For this review, take the finished solid that the model builds, in its own axes (mm). A direction names the side the tool comes from. Give positions to 0.01 mm unless a question says otherwise; leave off trailing zeros. Order: outer loops, then holes, each group sorted by start corner. A loop starts at its lowest first (then second) coordinate and runs counter-clockwise, first axis right, second up.
from build123d import *

# Parameters (mm, degrees)
SKETCH1_R             = 15
BOSS_EXTRUDE1_DEPTH   = 2
SKETCH2_W             = 12
SKETCH2_H             = 12
BOSS_EXTRUDE2_DEPTH   = 15
SKETCH3_R             = 2.5
CUT_EXTRUDE1_DEPTH    = 30.849623113
SKETCH4_R             = 10
BOSS_EXTRUDE3_DEPTH   = 30
FILLET1_R             = 5
SKETCH5_R             = 1.5
BOSS_EXTRUDE4_DEPTH   = 20
SKETCH7_R             = 0.5
BODY_MOVE_COPY2_ANGLE = 90


with BuildPart() as part:
    # Sketch1 → Boss-Extrude1 (new body)
    with BuildSketch(Plane.XY):
        Circle(SKETCH1_R)
    extrude(amount=-BOSS_EXTRUDE1_DEPTH)

    # Sketch2 → Boss-Extrude2 (add)
    with BuildSketch(Plane.XY):
        Rectangle(SKETCH2_W, SKETCH2_H)
    extrude(amount=BOSS_EXTRUDE2_DEPTH)

    # Sketch3 → Cut-Extrude1 (cut, through all)
    with BuildSketch(Plane(origin=(6, 0, 0), x_dir=(0, 0, -1), z_dir=(1, 0, 0))):
        with Locations(Location((-7.5, 0, 0), (0, 0, 90))):
            Circle(SKETCH3_R)
    extrude(amount=-CUT_EXTRUDE1_DEPTH, mode=Mode.SUBTRACT)

    # Sketch4 → Boss-Extrude3 (add)
    with BuildSketch(Plane(origin=(0, 0, -2), x_dir=(-1, 0, 0), z_dir=(0, 0, -1))):
        with Locations(Location((0, 0, 0), (0, 0, 180))):
            Circle(SKETCH4_R)
    extrude(amount=BOSS_EXTRUDE3_DEPTH)

    # Fillet1
    fillet1_edges = [part.edges().sort_by_distance(p)[0] for p in [
        (-10, 0, -32),
    ]]
    fillet(fillet1_edges, radius=FILLET1_R)

    # Sketch5 → Boss-Extrude4 (add)
    with BuildSketch(Plane(origin=(0, 0, -32), x_dir=(-1, 0, 0), z_dir=(0, 0, -1))):
        Circle(SKETCH5_R)
    extrude(amount=BOSS_EXTRUDE4_DEPTH)

    # Sketch7 → Loft2 section 0
    with BuildSketch(Plane(origin=(0, 0, -52), x_dir=(-1, 0, 0), z_dir=(0, 0, -1)), mode=Mode.PRIVATE) as loft2_s0:
        Circle(SKETCH7_R)
    loft([Vertex(0, 0, -54.75), loft2_s0.sketch])


with BuildPart() as part_1:
    # Body-Move/Copy1: moved
    add(part.part.moved(Location((0, 0, 52))))


with BuildPart() as part_2:
    # Body-Move/Copy2: moved
    add(part_1.part.rotate(Axis((0, 0, 0), (0, 1, 0)), BODY_MOVE_COPY2_ANGLE))


solid = part_2.part
1) We need section A-A on x = 59.5. Give the boundary of the cut face in (y, z).
Answer sheet:
outline: (-6, -6) - (-2.5, -6) - (-2.5, 6) - (-6, 6) - close; (2.5, -6) - (6, -6) - (6, 6) - (2.5, 6) - close
2) We need section B-B on x = 13.5. Give the boundary of the cut face in (y, z).
Answer sheet:
outline: circle Ø3 at (0, 0)
3) We need section D-D on x = 35. Give the boundary of the cut face in (y, z), then the cut area to 3 significant figures.
Answer sheet:
outline: circle Ø20 at (0, 0)
area: 314 mm2
4) Tool access review of faces 1 (the face through (59, 6, 0)), 2 (the face through (59, -6, 0)), 3 (the face through (59, 3, -6)), 4 (the face through (20, -1.2, 1.2)): name each direction out of +Z, -Z, +X, -X, +Y, -Y from which nothing blocks a thin tool from reaching the whole face with its end or side.
Answer sheet:
face 1: +Z, -Z, +X, +Y
face 2: +Z, -Z, +X, -Y
face 3: -Z, +X, +Y, -Y
face 4: -X
5) We need section C-C on y = -12.5. Give the boundary of the cut face in (x, z).
Answer sheet:
outline: (50, -8.29) - (52, -8.29) - (52, 8.29) - (50, 8.29) - close
6) Draft analysis for pull direction Y (two halves, no side actions). For faces 5 (the face through (59, 3, 6)), 6 (the face through (62, 0, 0)), 7 (the face through (10.14, 0.45, 1.43)), state which applies: +Y half, -Y half, draft (parallel to the pull), parting line (faces both ways), or undercut.
Answer sheet:
face 5: draft
face 6: undercut
face 7: parting line
7) To check wall thickness, follow line 1 (X direction, y = 0, z = 3); line 2 (X direction, y = 10.5, z = 9.5); line 3 (Z direction, x = 64, y = -4). State the ranges of each line that lie inside material, in increasing order.
Answer sheet:
line 1: x = 20 to 57, 62 to 67
line 2: x = 50 to 52
line 3: z = -6 to 6
8) Clearance check with flat-ended pins moving along their axes: pin 1 (6 mm diameter, centred on y = -3.5, z = 6, fed in from -X); pin 2 (9.5 mm diameter, centred on x = 62.5, z = 1, fed in from -Y); pin 3 (3 mm diameter, centred on x = 32.5, z = -1.5, fed in from +Y). State where each tip first meets the part, or that it passes through.
Answer sheet:
pin 1: stops at x = 20
pin 2: stops at y = -6
pin 3: stops at y = 10
